Verification items for the finished model (mm, model axes). A direction names the side the tool comes from. Give positions to 0.01 mm unless a question says otherwise; leave off trailing zeros. Write each loop counter-clockwise with the first axis right and the second up, starting at its lowest first coordinate (ties: lowest second). Pieces come first, ordered by that corner, then holes. Notation, with made-up numbers: (18.5, 18.5) -> (30.5, 18.5) arc R9 cw to (30.5, 30.5) -> close; hole circle Ø10 at (62.25, 60). An arc over 180 degrees is marked (long way). Use one line per item in the form item = value. Start each with the question number.
(1) Set-up check for faces 1 (the face through (44, 10, -259)), 2 (the face through (94.248, 4.93, -520.379)): record each of +Z, -Z, +X, -X, +Y, -Y from which the full face is reachable in a straight line by a thin tool's end or side.
(2) Release check for a two-part mould opening along Z. For faces 3 (the face through (44, 0, -259)), 4 (the face through (2.71, 4.93, -309.93)), 5 (the face through (-161.91, 4.93, -506.01)), 6 (the face through (-96.654, 4.93, -512.949)) record: pulls with the +Z half, pulls with the -Z half, needs draft (parallel to the pull), parting line crosses it, or undercut.
(3) Depth check by flat-ended pin: pin 1 Ø6 at (y, z) = (3.5, -708) entering from +X; pin 2 Ø1.5 at (y, z) = (6, -87) entering from -X; pin 3 Ø4 at (x, z) = (-45.56, -761.44) entering from -Y; pin 4 Ø3 at (y, z) = (1.5, -650) entering from +X. Enter the tip coordinate at first touch or a pass-through.
(4) Section check B-B, the plane z = -275.5. Record the cut outline in (x, y), plus the area to 3 significant figures.
(5) Section check C-C, the plane y = 6.5. State how many separate pieces and enclosed holes the cut face has, plus the area to 3 significant figures.
(6) Section check A-A, the plane z = 0. Record the cut outline in (x, y).
(7) Scan lines: L1, parallel to Z at x = 5, y = 6.5; L2, parallel to X at y = 7, z = 0; L3, parallel to X at y = 8.75, z = -253. Record each from-to range of solid material in increasing order.
(8) Section check D-D, the plane z = -427. Record the cut outline in (x, y).
from build123d import *

# Parameters (mm, degrees)
SKETCH2_R           = 250
SKETCH2_R_2         = 2.5
BOSS_EXTRUDE1_DEPTH = 10


with BuildPart() as part:
    # Sketch2 → Boss-Extrude1 (new body)
    with BuildSketch(Plane(origin=(0, 0, 0), x_dir=(1, 0, 0), z_dir=(0, 1, 0))):
        with BuildLine():
            Line((-32.627158959, 905.183764104), (-294.863184644, 95.498530059))
            ThreePointArc((-294.863184644, 95.498530059), (0, -309.942360613), (294.863184644, 95.498530059))
            Line((294.863184644, 95.498530059), (32.627158959, 905.183764104))
            ThreePointArc((32.627158959, 905.183764104), (28.995353361, 910.189981994), (23.11367445, 912.102593467))
            Line((23.11367445, 912.102593467), (-23.11367445, 912.102593467))
            ThreePointArc((-23.11367445, 912.102593467), (-28.995353361, 910.189981994), (-32.627158959, 905.183764104))
        make_face()
        Circle(SKETCH2_R, mode=Mode.SUBTRACT)
        with Locations((-184.210314713, 333.331115971)):
            Circle(SKETCH2_R_2, mode=Mode.SUBTRACT)
        with Locations((-137.992755162, 476.03338361)):
            Circle(SKETCH2_R_2, mode=Mode.SUBTRACT)
        with Locations((-91.775195611, 618.735651249)):
            Circle(SKETCH2_R_2, mode=Mode.SUBTRACT)
        with Locations((-45.557636061, 761.437918887)):
            Circle(SKETCH2_R_2, mode=Mode.SUBTRACT)
        with BuildLine():
            ThreePointArc((181.388362207, 251.321564848), (0, 309.942360613), (-181.388362207, 251.321564848))
            Line((-181.388362207, 251.321564848), (-9.513484509, 782.005898596))
            ThreePointArc((-9.513484509, 782.005898596), (0, 788.92472796), (9.513484509, 782.005898596))
            Line((9.513484509, 782.005898596), (181.388362207, 251.321564848))
        make_face(mode=Mode.SUBTRACT)
        with Locations((137.992755162, 476.03338361)):
            Circle(SKETCH2_R_2, mode=Mode.SUBTRACT)
        with Locations((184.210314713, 333.331115971)):
            Circle(SKETCH2_R_2, mode=Mode.SUBTRACT)
        with Locations((91.775195611, 618.735651249)):
            Circle(SKETCH2_R_2, mode=Mode.SUBTRACT)
        with Locations((45.557636061, 761.437918887)):
            Circle(SKETCH2_R_2, mode=Mode.SUBTRACT)
    extrude(amount=BOSS_EXTRUDE1_DEPTH)


solid = part.part
Completed:
q1.face_1 = +Z, -Z, +X, -X, +Y
q1.face_2 = +Y, -Y
q2.face_3 = needs draft
q2.face_4 = undercut
q2.face_5 = pulls with the -Z half
q2.face_6 = undercut
q3.pin_1 = 97.46
q3.pin_2 = -297.7
q3.pin_3 = through
q3.pin_4 = 115.76
q4.outline = (-236.57, 0) -> (-173.56, 0) -> (-173.56, 10) -> (-236.57, 10) -> close; (-142, 0) -> (142, 0) -> (142, 10) -> (-142, 10) -> close; (173.56, 0) -> (236.57, 0) -> (236.57, 10) -> (173.56, 10) -> close
q4.area = 4,100 mm²
q5.separate_pieces = 1
q5.enclosed_holes = 10
q5.area = 191,000 mm²
q6.outline = (-309.94, 0) -> (-250, 0) -> (-250, 10) -> (-309.94, 10) -> close; (250, 0) -> (309.94, 0) -> (309.94, 10) -> (250, 10) -> close
q7.L1 = -912.1 to -787.58, -309.9 to -249.95, 249.95 to 309.9
q7.L2 = -309.94 to -250, 250 to 309.94
q7.L3 = -243.85 to -180.84, -179.04 to 179.04, 180.84 to 243.85
q8.outline = (-187.5, 0) -> (-124.49, 0) -> (-124.49, 10) -> (-187.5, 10) -> close; (124.49, 0) -> (187.5, 0) -> (187.5, 10) -> (124.49, 10) -> close
